The figure shows three views and two pictorial views of one solid part (mm, origin at its lowest corner). Answer the questions. A direction names the side the tool comes from. Coordinates: 2 decimals unless noted, no trailing zeros. Loops run counter-clockwise (first coordinate to the right, second up) from the corner with the lowest first, then second, coordinate; pieces in that order, holes last. Notation, with made-up numbers: M 26,78 L 35,78 A29 cw 35,111 Z; hole C 86,52 d6. An arc over 180 degrees is marked long. One line per item, written item: value. Start each with the question number.
1. Determine the mould class of the marked faces 1, 2 and 3 for opening direction Y: +Y half, -Y half, draft (parallel to the pull), parting line (faces both ways), or undercut.
2. Flat-ended cylindrical pins translate along their axes: pin 1 (1 mm diameter, centred on y = 84, z = 9, fed in from +X); pin 2 (3 mm diameter, centred on x = 30, z = 16.5, fed in from +Y); pin 3 (6.5 mm diameter, centred on x = 18, z = 14.5, fed in from -Y); pin 4 (1 mm diameter, centred on y = 17.5, z = 15.5, fed in from -X) (1 decimal). Find the tip coordinate at first contact, or state that the pin passes through.
3. The part is cut by section D-D (x = 6). Write down the section's boundary in (y, z), then the cut area to 3 significant figures.
4. Consider probe 1 along Y at (x, z) = (7.5, 2.5); probe 2 along X at (y, z) = (21, 8) (1 decimal); probe 3 along X at (y, z) = (79, 9.25) (1 decimal). Determine where each line is inside the solid, lowest interval first.
5. The part is cut by section B-B (y = 53). Write down the section's boundary in (x, z) (1 decimal).
6. For the marked faces 4, 5, 6, 7 and 8, determine the directions among +Z, -Z, +X, -X, +Y, -Y from which every point of the face is accessible in a straight line to the end or side of a thin tool.
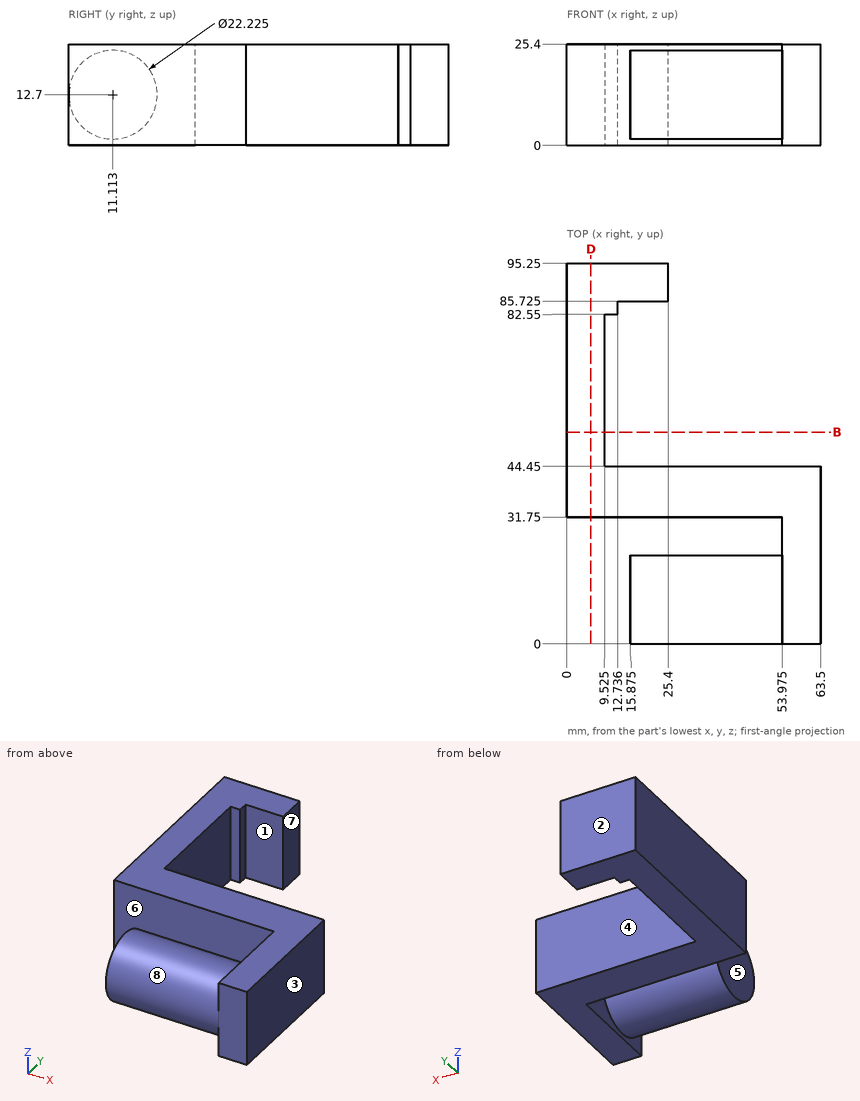
Answer block:
1. face 1: undercut
1. face 2: +Y half
1. face 3: draft
2. pin 1: stops at x = 12.74
2. pin 2: stops at y = 44.45
2. pin 3: stops at y = 0
2. pin 4: stops at x = 15.9
3. outline: M 31.75,0 L 95.25,0 L 95.25,25.4 L 31.75,25.4 Z
3. area: 1,610 mm2
4. probe 1: y = 31.75 to 95.25
4. probe 2: x = 15.9 to 63.5
4. probe 3: x = 0 to 9.5
5. outline: M 0,0 L 9.5,0 L 9.5,25.4 L 0,25.4 Z
6. face 4: +Z, -Z, +X
6. face 5: +Z, -Z, -X, -Y
6. face 6: +Z, -Z, -X
6. face 7: +Z, -Z, +X, +Y
6. face 8: -X
